```python
from build123d import *

# Parameters (mm, degrees)
BOSS_EXTRUDE1_DEPTH = 3
CUT_EXTRUDE1_REACH  = 138.82
CUT_EXTRUDE2_DEPTH  = 1
CUT_EXTRUDE3_DEPTH  = 3


with BuildPart() as part:
    # Sketch3 → Boss-Extrude1 (new body)
    with BuildSketch(Plane(origin=(0, 0, 0), x_dir=(1, 0, 0), z_dir=(0, 1, 0))):
        with BuildLine():
            Line((131.37466785, -33.834747513), (131.37466785, -26.093767651))
            Line((131.37466785, -26.093767651), (-8.62533215, -26.093767651))
            Line((-8.62533215, -26.093767651), (-8.62533215, -33.834747513))
            ThreePointArc((-8.62533215, -33.834747513), (-7.746652493, -35.956067857), (-5.62533215, -36.834747513))
            Line((-5.62533215, -36.834747513), (-5.431022837, -36.834747513))
            ThreePointArc((-5.431022837, -36.834747513), (-3.945556452, -37.165616778), (-2.74094445, -38.095667731))
            Line((-2.74094445, -38.095667731), (125.49028015, -38.095667731))
            ThreePointArc((125.49028015, -38.095667731), (126.694892152, -37.165616778), (128.180358538, -36.834747513))
            Line((128.180358538, -36.834747513), (128.37466785, -36.834747513))
            ThreePointArc((128.37466785, -36.834747513), (130.495988194, -35.956067857), (131.37466785, -33.834747513))
        make_face()
    extrude(amount=BOSS_EXTRUDE1_DEPTH)

    # Sketch4 → Cut-Extrude1 (cut, up to next)
    with BuildSketch(Plane(origin=(0, 3, 0), x_dir=(1, 0, 0), z_dir=(0, 1, 0)), mode=Mode.PRIVATE) as cut_extrude1_sk1:
        with BuildLine():
            ThreePointArc((81.109797099, -31.496885933), (79.509797099, -33.096885933), (81.109797099, -34.696885933))
            ThreePointArc((81.109797099, -34.696885933), (82.709797099, -33.096885933), (81.109797099, -31.496885933))
        make_face()
    cut_extrude1_tool1 = extrude(cut_extrude1_sk1.sketch, amount=-CUT_EXTRUDE1_REACH, mode=Mode.PRIVATE) & part.part
    # Sketch4 → Cut-Extrude1 (cut, up to next)
    with BuildSketch(Plane(origin=(0, 3, 0), x_dir=(1, 0, 0), z_dir=(0, 1, 0)), mode=Mode.PRIVATE) as cut_extrude1_sk2:
        with BuildLine():
            ThreePointArc((41.109797099, -31.496885933), (39.509797099, -33.096885933), (41.109797099, -34.696885933))
            ThreePointArc((41.109797099, -34.696885933), (42.709797099, -33.096885933), (41.109797099, -31.496885933))
        make_face()
    cut_extrude1_tool2 = extrude(cut_extrude1_sk2.sketch, amount=-CUT_EXTRUDE1_REACH, mode=Mode.PRIVATE) & part.part
    add(cut_extrude1_tool1.solids().sort_by_distance((81.109797, 3, 33.096886))[0], mode=Mode.SUBTRACT)
    add(cut_extrude1_tool2.solids().sort_by_distance((41.109797, 3, 33.096886))[0], mode=Mode.SUBTRACT)

    # Sketch5 → Cut-Extrude2 (cut)
    with BuildSketch(Plane.XZ):
        with BuildLine():
            Line((12.809243061, 32.25429666), (12.495140497, 32.25429666))
            add(Edge.make_bspline(
                [(12.495140497, 32.25429666), (12.49718765, 32.295967547), (12.501208204, 32.377808062), (12.520036494, 32.497131968), (12.546977371, 32.611186767), (12.585068825, 32.719056681), (12.632375103, 32.821695488), (12.68910513, 32.918695504), (12.75629898, 33.009686693), (12.832505715, 33.093825536), (12.915274354, 33.171013107), (13.004580293, 33.23766835), (13.09842532, 33.293986021), (13.196524719, 33.341067263), (13.299985283, 33.376407109), (13.407868141, 33.402628748), (13.520647277, 33.418405094), (13.597487299, 33.42010088), (13.636566779, 33.420963326)],
                knots=[0, 0, 0, 0, 1.10065271, 2.161652631, 3.183658789, 4.190468796, 5.17591951, 6.163126047, 7.15150782, 8.156236427, 9.156009102, 10.134482811, 11.092018607, 12.041330605, 13.001268258, 13.972401359, 14.968799086, 16, 16, 16, 16], degree=3))
            add(Edge.make_bspline(
                [(13.636566779, 33.420963326), (13.674944853, 33.42006487), (13.750356398, 33.418299435), (13.860418413, 33.403138406), (13.965195707, 33.379392814), (14.064483474, 33.346077398), (14.157489538, 33.30129297), (14.244912583, 33.247495432), (14.327793393, 33.1852756), (14.402400177, 33.112021787), (14.470908256, 33.033819402), (14.530010511, 32.950331499), (14.580623675, 32.864102213), (14.622811355, 32.774474012), (14.653867494, 32.680602983), (14.677445702, 32.58385578), (14.690773115, 32.483230969), (14.692818539, 32.415124414), (14.693858446, 32.380498583)],
                knots=[0, 0, 0, 0, 1.111607364, 2.184268762, 3.212621178, 4.221274766, 5.211760367, 6.196651075, 7.1921475, 8.207485113, 9.220403448, 10.201281604, 11.166441695, 12.114753415, 13.065576456, 14.026450734, 14.996634279, 16, 16, 16, 16], degree=3))
            add(Edge.make_bspline(
                [(14.693858446, 32.380498583), (14.692171801, 32.331748773), (14.688828109, 32.235104645), (14.659972407, 32.092900288), (14.61539031, 31.954995228), (14.561317281, 31.844016176), (14.506696713, 31.755039283), (14.458516917, 31.681123642), (14.400864565, 31.602297225), (14.334267151, 31.517766116), (14.259729345, 31.427271746), (14.176714677, 31.33077698), (14.084588987, 31.229306675), (14.019930805, 31.160000862), (13.986426555, 31.124088326)],
                knots=[0, 0, 0, 0, 1.184203166, 2.347625244, 3.513805382, 4.700623107, 5.337941753, 6.051866363, 6.845199593, 7.711357327, 8.668078039, 9.695487809, 10.805859518, 12, 12, 12, 12], degree=3))
            Line((13.986426555, 31.124088326), (13.110725433, 30.190194095))
            Line((13.110725433, 30.190194095), (14.738730241, 30.190194095))
            Line((14.738730241, 30.190194095), (14.738730241, 29.831219737))
            Line((14.738730241, 29.831219737), (12.360525113, 29.831219737))
            Line((12.360525113, 29.831219737), (13.717896908, 31.279737365))
            add(Edge.make_bspline(
                [(13.717896908, 31.279737365), (13.750944794, 31.314235671), (13.814423021, 31.380499858), (13.904205598, 31.477242818), (13.984844587, 31.566992359), (14.056861979, 31.649578907), (14.118695485, 31.726210475), (14.173567717, 31.794405179), (14.217533308, 31.857159629), (14.265248703, 31.929900243), (14.311462685, 32.01871256), (14.351175041, 32.127246249), (14.375389889, 32.238973502), (14.378294725, 32.314475539), (14.379755882, 32.352453711)],
                knots=[0, 0, 0, 0, 1.329631726, 2.553950428, 3.673215718, 4.687767853, 5.603093632, 6.413772471, 7.123043292, 7.734684054, 8.834405432, 9.900288307, 10.943827018, 12, 12, 12, 12], degree=3))
            add(Edge.make_bspline(
                [(14.379755882, 32.352453711), (14.37912014, 32.376335109), (14.377867214, 32.42340076), (14.366809516, 32.492406519), (14.35009901, 32.558971332), (14.326153752, 32.623299952), (14.294547012, 32.684745604), (14.256073632, 32.743383084), (14.211683569, 32.800072049), (14.160332299, 32.853225347), (14.103920779, 32.901906553), (14.04432653, 32.945030638), (13.981276426, 32.981069749), (13.915036303, 33.010613246), (13.845790834, 33.033788627), (13.773406089, 33.049847207), (13.698082073, 33.059929691), (13.646648577, 33.061293862), (13.620440978, 33.061988967)],
                knots=[0, 0, 0, 0, 0.991446411, 1.95395049, 2.89581595, 3.838931463, 4.798493298, 5.75982156, 6.748411868, 7.785213223, 8.824556874, 9.840280684, 10.836137867, 11.835679398, 12.848801643, 13.863922112, 14.911575587, 16, 16, 16, 16], degree=3))
            add(Edge.make_bspline(
                [(13.620440978, 33.061988967), (13.593070145, 33.061273935), (13.539318349, 33.05986973), (13.460399316, 33.050047066), (13.385113539, 33.033101225), (13.313271636, 33.009924551), (13.24475205, 32.980466002), (13.179888006, 32.943774257), (13.118825117, 32.899990764), (13.061448593, 32.850350208), (13.008584614, 32.795082607), (12.962137738, 32.733472644), (12.921553724, 32.666645228), (12.886144491, 32.594780678), (12.857388801, 32.517226898), (12.83541565, 32.434259193), (12.818028803, 32.346237811), (12.812220283, 32.285452727), (12.809243061, 32.25429666)],
                knots=[0, 0, 0, 0, 1.031018746, 2.02475058, 2.990194455, 3.934040569, 4.864654155, 5.795059489, 6.735614925, 7.690564532, 8.649604399, 9.611025574, 10.590972636, 11.591080095, 12.624614302, 13.701020113, 14.821632451, 16, 16, 16, 16], degree=3))
        make_face()
    extrude(amount=-CUT_EXTRUDE2_DEPTH, mode=Mode.SUBTRACT)

    # Sketch6 → Cut-Extrude3 (cut)
    with BuildSketch(Plane(origin=(0, 3, 0), x_dir=(1, 0, 0), z_dir=(0, 1, 0))):
        with BuildLine():
            Line((5.852113338, -30.785571201), (-4.565790678, -30.785571201))
            ThreePointArc((-4.565790678, -30.785571201), (-5.98000424, -31.371357639), (-6.565790678, -32.785571201))
            Line((-6.565790678, -32.785571201), (-6.565790678, -34.477380503))
            ThreePointArc((-6.565790678, -34.477380503), (-5.98000424, -35.891594066), (-4.565790678, -36.477380503))
            Line((-4.565790678, -36.477380503), (5.852113338, -36.477380503))
            ThreePointArc((5.852113338, -36.477380503), (7.266326901, -35.891594066), (7.852113338, -34.477380503))
            Line((7.852113338, -34.477380503), (7.852113338, -32.785571201))
            ThreePointArc((7.852113338, -32.785571201), (7.266326901, -31.371357639), (5.852113338, -30.785571201))
        make_face()
    extrude(amount=-CUT_EXTRUDE3_DEPTH, mode=Mode.SUBTRACT)


solid = part.part
```
Read the model definition and answer for the solid it produces. Units are mm, in the model's axes. A direction names the side the tool comes from. Give positions to 0.01 mm unless a question says otherwise; leave off trailing zeros. Write each loop counter-clockwise with the first axis right and the second up, starting at its lowest first coordinate (ties: lowest second). Pieces come first, ordered by that corner, then holes. Notation, with made-up numbers: M -5.5,77.5 L 10.5,77.5 A24 ccw 10.5,89.5 Z; hole C 21.25,-24 d5. An arc over 180 degrees is marked long. Put each result on its own line as item: value. Start each with the question number.
1. Consider line 1 along X through (y, z) = (2.05, 31.75); line 2 along X through (y, z) = (2.65, 34); line 3 along X through (y, z) = (0.95, 31). Determine where each line is inside the solid, lowest interval first.
2. Which of the six approach directions +Z, -Z, +X, -X, +Y, -Y give full straight-line access (tool end or side, diameter ignored) to faces 1 (the flat face through (1, 2, 30.786)), 2 (the cylindrical face through (126.675, 1.479, 37.175))?
3. The part is cut by section A-A, the plane y = 2. Give the vertices of the cut face in (x, z), and give its area (3 significant figures).
4. For a pull along Z with two mould halves and no side action, classify faces 3 (the flat face through (60, 3, 32)), 4 (the flat face through (60, 1, 38.096)), 5 (the flat face through (1, 2, 36.477)) as released by +Z, released by -Z, zero draft, split by the parting line, or undercut.
Final values:
1. line 1: x = -8.63 to -6.28, 7.56 to 40.25, 41.97 to 80.25, 81.97 to 131.37
1. line 2: x = -8.62 to -6.57, 7.85 to 39.79, 42.43 to 79.79, 82.43 to 131.37
1. line 3: x = -8.63 to -5.47, 6.75 to 13.46, 13.87 to 131.37
2. face 1: +Y, -Y
2. face 2: +Z, +X, +Y, -Y
3. outline: M -8.63,26.09 L 131.37,26.09 L 131.37,33.83 A3 ccw 128.37,36.83 L 128.18,36.83 A3.5 cw 125.49,38.1 L -2.74,38.1 A3.5 cw -5.43,36.83 L -5.63,36.83 A3 ccw -8.63,33.83 Z; hole M -6.57,32.79 A2 ccw -4.57,30.79 L 5.85,30.79 A2 ccw 7.85,32.79 L 7.85,34.48 A2 ccw 5.85,36.48 L -4.57,36.48 A2 ccw -6.57,34.48 Z; hole C 41.11,33.1 d3.2; hole C 81.11,33.1 d3.2
3. area: 1,570 mm²
4. face 3: zero draft
4. face 4: released by +Z
4. face 5: undercut
